Verification items for this drawing (mm, ordinates from the low corner). Coordinates: 2 decimals unless noted, no trailing zeros. Write each loop counter-clockwise with the first axis right and the second up, starting at its lowest first coordinate (ties: lowest second). Pieces come first, ordered by that corner, then holes. Notation, with made-up numbers: (70.25, 52.5) -> (93.25, 52.5) arc R19 ccw to (93.25, 89.5) -> close; hole circle Ø1 at (62, 26). An arc over 180 degrees is marked (long way). Use CSV: the item, a comma, the result in double quotes.
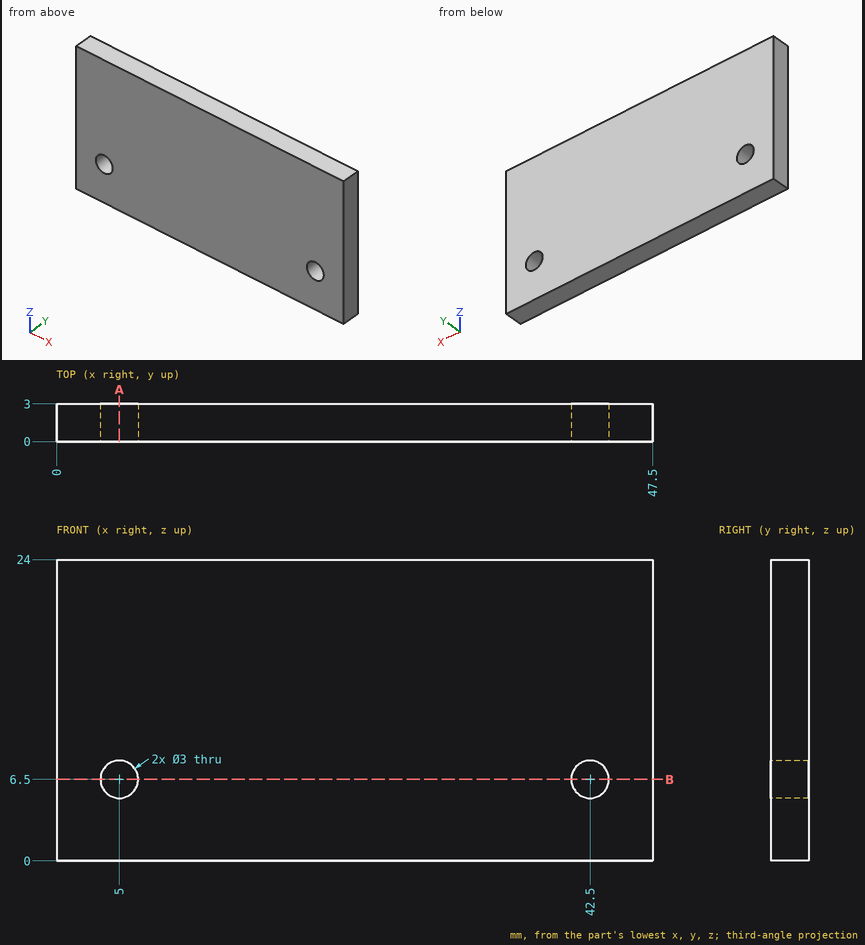
1) Cross-section at B-B (z = 6.5). Record the boundary of the cut face in (x, y), plus the area to 4 significant figures.
Return value:
outline,"(0, 0) -> (3.5, 0) -> (3.5, 3) -> (0, 3) -> close; (6.5, 0) -> (41, 0) -> (41, 3) -> (6.5, 3) -> close; (44, 0) -> (47.5, 0) -> (47.5, 3) -> (44, 3) -> close"
area,"124.5 mm2"
2) Scan lines: L1, parallel to X at y = 1.5, z = 6.5; L2, parallel to Z at x = 42.5, y = 1.55; L3, parallel to X at y = 1.1, z = 7.25. Record each from-to range of solid material in increasing order.
Return value:
L1,"0 to 3.5, 6.5 to 41, 44 to 47.5"
L2,"0 to 5, 8 to 24"
L3,"0 to 3.7, 6.3 to 41.2, 43.8 to 47.5"
3) Cross-section at A-A (x = 5). Record the boundary of the cut face in (y, z), plus the area to 3 significant figures.
Return value:
outline,"(0, 0) -> (3, 0) -> (3, 5) -> (0, 5) -> close; (0, 8) -> (3, 8) -> (3, 24) -> (0, 24) -> close"
area,"63.0 mm2"
